from build123d import *

# Parameters (mm, degrees)
SKETCH_2_R        = 0.25
EXTRUDE_1_DEPTH   = 9
EXTRUDE_1_2_DEPTH = 9
EXTRUDE_1_3_DEPTH = 9
EXTRUDE_2_DEPTH   = 1.5
SKETCH_4_R        = 4
EXTRUDE_3_DEPTH   = 0.4
SKETCH_5_R        = 3.3
EXTRUDE_4_DEPTH   = 3


with BuildPart() as part:
    # Sketch 2 → Extrude 1 (new body)
    with BuildSketch(Plane(origin=(0, 0, 0), x_dir=(1, 0, 0), z_dir=(0, 1, 0))):
        with Locations(Location((-1.27, 0, 0), (0, 0, 270))):
            Circle(SKETCH_2_R)
    extrude(amount=EXTRUDE_1_DEPTH)



with BuildPart() as body_2:
    # Sketch 2 → Extrude 1 2 (new body)
    with BuildSketch(Plane(origin=(0, 0, 0), x_dir=(1, 0, 0), z_dir=(0, 1, 0))):
        with Locations(Location((0.630957819, 1.102176134, 0), (0, 0, 270))):
            Circle(SKETCH_2_R)
    extrude(amount=EXTRUDE_1_2_DEPTH)


with BuildPart() as body_3:
    # Sketch 2 → Extrude 1 3 (new body)
    with BuildSketch(Plane(origin=(0, 0, 0), x_dir=(1, 0, 0), z_dir=(0, 1, 0))):
        with Locations(Location((0.630957819, -1.102176134, 0), (0, 0, 270))):
            Circle(SKETCH_2_R)
    extrude(amount=EXTRUDE_1_3_DEPTH)


with BuildPart() as part_1:
    add(part.part)

    add(body_2.part)  # Extrude 2 merges body 2

    add(body_3.part)  # Extrude 2 merges body 3
    # Sketch 3 → Extrude 2 (add)
    with BuildSketch(Plane(origin=(0, 9, 0), x_dir=(1, 0, 0), z_dir=(0, 1, 0))):
        with BuildLine():
            Line((-4.247340401, 0), (-4.493274572, 0.245934171))
            ThreePointArc((-4.493274572, 0.245934171), (4.5, 0), (-4.493274572, -0.245934171))
            Line((-4.493274572, -0.245934171), (-4.247340401, 0))
        make_face()
    extrude(amount=EXTRUDE_2_DEPTH)

    # Sketch 4 → Extrude 3 (add)
    with BuildSketch(Plane(origin=(0, 10.5, 0), x_dir=(1, 0, 0), z_dir=(0, 1, 0))):
        with Locations(Location((0, 0, 0), (0, 0, 270))):
            Circle(SKETCH_4_R)
    extrude(amount=EXTRUDE_3_DEPTH)

    # Sketch 5 → Extrude 4 (add)
    with BuildSketch(Plane(origin=(0, 10.9, 0), x_dir=(1, 0, 0), z_dir=(0, 1, 0))):
        with Locations(Location((0, 0, 0), (0, 0, 270))):
            Circle(SKETCH_5_R)
    extrude(amount=EXTRUDE_4_DEPTH)


solid = part_1.part
Work out the finished part from the listing and answer in its coordinate system (mm). A direction names the side the tool comes from. Round coordinates to 2 decimals unless told otherwise and drop trailing zeros. Loops run counter-clockwise (first coordinate to the right, second up) from the corner with the lowest first, then second, coordinate; pieces in that order, holes last. Notation, with made-up numbers: (34, -17) -> (72, -17) arc R8 cw to (72, -2) -> close; hole circle Ø8 at (-7, 28). An arc over 180 degrees is marked (long way). Use one line per item in the form item = value.
(1) Find section C-C on y = 7.75. Give the vertices of the cut face in (x, z), then the cut area to 3 significant figures.
Answer list:
outline = circle Ø0.5 at (-1.27, 0); circle Ø0.5 at (0.63, -1.1); circle Ø0.5 at (0.63, 1.1)
area = 0.589 mm2
(2) Find section D-D on y = 11.75. Give the vertices of the cut face in (x, z), then the cut area to 3 significant figures.
Answer list:
outline = circle Ø6.6 at (0, 0)
area = 34.2 mm2
(3) Straight lines are drawn through the part: line 1 (Y direction, x = -1.25, z = 3); line 2 (Z direction, x = -1.25, y = 4.25); line 3 (Y direction, x = 0.25, z = 3.75). For each, find the intervals that lie inside material, in ascending order.
Answer list:
line_1 = 9 to 13.9
line_2 = -0.25 to 0.25
line_3 = 9 to 10.9
(4) Find section A-A on x = 0. Give the vertices of the cut face in (y, z).
Answer list:
outline = (9, -4.5) -> (10.5, -4.5) -> (10.5, -4) -> (10.9, -4) -> (10.9, -3.3) -> (13.9, -3.3) -> (13.9, 3.3) -> (10.9, 3.3) -> (10.9, 4) -> (10.5, 4) -> (10.5, 4.5) -> (9, 4.5) -> close
(5) Flat-ended cylindrical pins translate along their axes: P1, Ø2.5, axis at x = -2, z = -2, coming from the -Y side; P2, Ø3, axis at y = 2.5, z = -1, coming from the +X side. Find the tip coordinate at first contact, or state that the pin passes through.
Answer list:
P1 = 9
P2 = 0.88
(6) A tool of negligible diameter and unlimited length cuts with its end or side. For faces 3 (the flat face through (3, 10.9, -2)), 4 (the flat face through (0, 13.9, 0)), from which of +Z, -Z, +X, -X, +Y, -Y can it reach the whole face along a straight path? Write none if from no direction.
Answer list:
face_3 = +Y
face_4 = +Z, -Z, +X, -X, +Y
(7) For a pull along Z with two mould halves and no side action, classify faces 1 (the cylindrical face through (4.496, 9.74, -0.194)), 2 (the flat face through (3, 10.5, 3)) as released by +Z, released by -Z, zero draft, split by the parting line, or undercut.
Answer list:
face_1 = split by the parting line
face_2 = zero draft
(8) Find section B-B on z = 2.75. Give the vertices of the cut face in (x, y).
Answer list:
outline = (-3.56, 9) -> (3.56, 9) -> (3.56, 10.5) -> (2.9, 10.5) -> (2.9, 10.9) -> (1.82, 10.9) -> (1.82, 13.9) -> (-1.82, 13.9) -> (-1.82, 10.9) -> (-2.9, 10.9) -> (-2.9, 10.5) -> (-3.56, 10.5) -> close
